Build history of the part. All positions in model axes, mm. Give positions to 0.01 mm unless a question says otherwise; leave off trailing zeros. Order: outer loops, then holes, each group sorted by start corner. A loop starts at its lowest first (then second) coordinate and runs counter-clockwise, first axis right, second up. Notation, with made-up numbers: (0, 9.5) - (46, 9.5) arc R24 cw to (46, 34.5) - close; hole circle Ø8 at (-35.75, -29). An arc over 180 degrees is marked (long way). One line per item, written item: value.
```python
from build123d import *

# Parameters (mm, degrees)
SKETCH_1_R             = 6
EXTRUDE_1_DEPTH        = 60
FILLET_1_R             = 6
CHAMFER_1_SIZE         = 0.5
HOLE_WIZARD_M4_1_D     = 3.3
HOLE_WIZARD_M4_1_DEPTH = 11.5
HOLE_WIZARD_M4_1_TIP   = 0.991420021


with BuildPart() as part:
    # 草圖1 → 伸長1 (new body)
    with BuildSketch(Plane.XY):
        Circle(SKETCH_1_R)
    extrude(amount=EXTRUDE_1_DEPTH)

    # 圓角1
    fillet_1_edges = [part.edges().sort_by_distance(p)[0] for p in [
        (-6, 0, 0),
    ]]
    fillet(fillet_1_edges, radius=FILLET_1_R)

    # 導角1
    chamfer_1_edges = [part.edges().sort_by_distance(p)[0] for p in [
        (-6, 0, 60),
    ]]
    chamfer(chamfer_1_edges, length=CHAMFER_1_SIZE)

    # M4 螺紋孔1
    with Locations(Plane.XY.offset(60)):
        with Locations((0, 0)):
            Hole(HOLE_WIZARD_M4_1_D / 2, depth=HOLE_WIZARD_M4_1_DEPTH)
            with Locations((0, 0, -(HOLE_WIZARD_M4_1_DEPTH + HOLE_WIZARD_M4_1_TIP / 2))):  # 118° drill point
                Cone(0, HOLE_WIZARD_M4_1_D / 2, HOLE_WIZARD_M4_1_TIP, mode=Mode.SUBTRACT)


solid = part.part
```
(1) Pin check, flat tips, straight feed: P1, Ø5, axis at y = 4, z = 13, coming from the -X side; P2, Ø6, axis at x = 4.5, z = 24.5, coming from the +Y side; P3, Ø4, axis at y = -4.5, z = 45.5, coming from the +X side. Stop position of each tip, or through.
Completed:
P1: x = -5.81
P2: y = 5.81
P3: x = 5.45
(2) Pull direction X, two halves, no side cores. Call faces 1 (the face through (-0.1, -0.3, 47.7)), 2 (the face through (-6, 0, 32)), 3 (the face through (-1.3, 1.3, 60)), 4 (the face through (1.216, 1.115, 54.17)): +X half, -X half, draft (parallel to the pull), parting line (faces both ways), or undercut.
Completed:
face 1: undercut
face 2: parting line
face 3: draft
face 4: undercut
(3) Drill centre lines: line 1 (Y direction, x = 0, z = 52.75); line 2 (Z direction, x = 2.25, y = 3); line 3 (Y direction, x = 2.5, z = 40.5). Where is each one in solid material? Low to high.
Completed:
line 1: -6 to -1.65, 1.65 to 6
line 2: 1.32 to 60
line 3: -5.45 to 5.45
(4) Slice it at A-A, the plane z = 54. Give the cut face in (x, y).
Completed:
outline: circle Ø12 at (0, 0); hole circle Ø3.3 at (0, 0)
(5) Slice it at B-B, the plane z = 26.5. Give the cut face in (x, y).
Completed:
outline: circle Ø12 at (0, 0)
